```python
from build123d import *

# Parameters (mm, degrees)
SKETCH1_W           = 88.5
SKETCH1_H           = 88.5
SKETCH1_R           = 2
BOSS_EXTRUDE1_DEPTH = 4.6
SKETCH2_R           = 2.5
BOSS_EXTRUDE2_DEPTH = 3
SKETCH3_W           = 88.5
SKETCH3_H           = 88.5
BOSS_EXTRUDE3_DEPTH = 1
FILLET1_R           = 2
SKETCH4_W           = 2.25
SKETCH4_H           = 2.25
CUT_EXTRUDE1_DEPTH  = 4
SKETCH5_W           = 72.5
SKETCH5_H           = 72.5
CUT_EXTRUDE2_DEPTH  = 4


with BuildPart() as part:
    # Sketch1 → Boss-Extrude1 (new body)
    with BuildSketch(Plane.XY):
        with Locations((-44.25, -44.25)):
            Rectangle(SKETCH1_W, SKETCH1_H)
        with Locations((-86.25, -86.25)):
            Circle(SKETCH1_R, mode=Mode.SUBTRACT)
        with Locations((-2.25, -86.25)):
            Circle(SKETCH1_R, mode=Mode.SUBTRACT)
        with Locations((-2.25, -2.25)):
            Circle(SKETCH1_R, mode=Mode.SUBTRACT)
        with Locations((-86.25, -2.25)):
            Circle(SKETCH1_R, mode=Mode.SUBTRACT)
    extrude(amount=BOSS_EXTRUDE1_DEPTH)

    # Sketch2 → Boss-Extrude2 (add)
    with BuildSketch(Plane.XY.offset(4.6)):
        with Locations((-5, -83.5)):
            Circle(SKETCH2_R)
        with Locations((-83.5, -83.5)):
            Circle(SKETCH2_R)
        with Locations((-5, -5)):
            Circle(SKETCH2_R)
        with Locations((-83.5, -5)):
            Circle(SKETCH2_R)
    extrude(amount=BOSS_EXTRUDE2_DEPTH)

    # Sketch3 → Boss-Extrude3 (add)
    with BuildSketch(Plane.XY.offset(4.6)):
        with Locations((-44.25, -44.25)):
            Rectangle(SKETCH3_W, SKETCH3_H)
    extrude(amount=BOSS_EXTRUDE3_DEPTH)

    # Fillet1
    fillet1_edges = [part.edges().sort_by_distance(p)[0] for p in [
        (0, 0, 2.8),
        (0, -88.5, 2.8),
        (-88.5, -88.5, 2.8),
        (-88.5, 0, 2.8),
        (-88.5, -44.25, 5.6),
        (-44.25, -88.5, 5.6),
        (0, -44.25, 5.6),
        (-44.25, 0, 5.6),
    ]]
    fillet(fillet1_edges, radius=FILLET1_R)

    # Sketch4 → Cut-Extrude1 (cut)
    with BuildSketch(Plane(origin=(0, 0, 0), x_dir=(-1, 0, 0), z_dir=(0, 0, -1))):
        with Locations((87.375, -87.375)):
            Rectangle(SKETCH4_W, SKETCH4_H)
        with Locations((1.125, -87.375)):
            Rectangle(SKETCH4_W, SKETCH4_H)
        with Locations((87.375, -1.125)):
            Rectangle(SKETCH4_W, SKETCH4_H)
        with Locations((1.125, -1.125)):
            Rectangle(SKETCH4_W, SKETCH4_H)
    extrude(amount=-CUT_EXTRUDE1_DEPTH, mode=Mode.SUBTRACT)

    # Sketch5 → Cut-Extrude2 (cut)
    with BuildSketch(Plane.XY.offset(5.6)):
        with Locations((-44.25, -44.25)):
            Rectangle(SKETCH5_W, SKETCH5_H)
    extrude(amount=-CUT_EXTRUDE2_DEPTH, mode=Mode.SUBTRACT)


solid = part.part
```
Geometry: final body of the model. Coordinates: model frame, mm. A direction names the side the tool comes from. Round coordinates to 2 decimals unless told otherwise and drop trailing zeros. Write each loop counter-clockwise with the first axis right and the second up, starting at its lowest first coordinate (ties: lowest second). Pieces come first, ordered by that corner, then holes. Notation, with made-up numbers: (-26.5, 29) -> (-19.5, 29) arc R24 ccw to (-19.5, 49) -> close; hole circle Ø4 at (30, 3). An arc over 180 degrees is marked (long way). Return JSON: item names as keys, results as strings.
Q1. Section A-A on y = -13. Return the cut outline in (x, z).
From the geometry:
{"outline": "(-88.5, 0) -> (0, 0) -> (0, 3.6) arc R2 ccw to (-2, 5.6) -> (-8, 5.6) -> (-8, 1.6) -> (-80.5, 1.6) -> (-80.5, 5.6) -> (-86.5, 5.6) arc R2 ccw to (-88.5, 3.6) -> close"}
Q2. Set-up query: faces 1 (the flat face through (-45, -80.5, 4)), 2 (the flat face through (-45, -88.5, 2)), 3 (the flat face through (-88, -1, 4)), 4 (the flat face through (0, -45, 2)), 5 (the flat face through (-2, -86, 4.6)). Return all of +Z, -Z, +X, -X, +Y, -Y with unobstructed straight access to the full face (end or side cutting, diameter ignored); none if empty.
From the geometry:
{"face 1": "+Z", "face 2": "+Z, -Z, +X, -X, -Y", "face 3": "-Z, -X, +Y", "face 4": "+Z, -Z, +X, +Y, -Y", "face 5": "-Z"}
Q3. Ray query, line 1 (Y direction, x = -77.5, z = 3.75); line 2 (X direction, y = -15.5, z = 4); line 3 (Z direction, x = -74, y = -34.5). Return the intervals inside material, ascending.
From the geometry:
{"line 1": "-88.49 to -80.5, -8 to -0.01", "line 2": "-88.46 to -80.5, -8 to -0.04", "line 3": "0 to 1.6"}
Q4. Mould query, pull axis Y, two halves, no side actions, for faces 6 (the cylindrical face through (-87.93, -43.66, 5)), 7 (the flat face through (-80.5, -45, 4)), 8 (the cylindrical face through (-43.66, -87.93, 5)). Classes: +Y half, -Y half, draft (parallel to the pull), parting line (faces both ways), or undercut.
From the geometry:
{"face 6": "draft", "face 7": "undercut", "face 8": "-Y half"}
Q5. First-contact query: pin 1 Ø3 at (x, y) = (-86.25, -2.25) entering from -Z; pin 2 Ø3 at (x, z) = (-53, 4) entering from -Y; pin 3 Ø1 at (x, y) = (-50.5, -68.5) entering from +Z; pin 4 Ø1.5 at (y, z) = (-24, 4.5) entering from -X. Flat tips, straight axial feed; report the tip coordinate or a pass-through.
From the geometry:
{"pin 1": "z = 4.6", "pin 2": "y = -88.5", "pin 3": "z = 1.6", "pin 4": "x = -88.49"}
